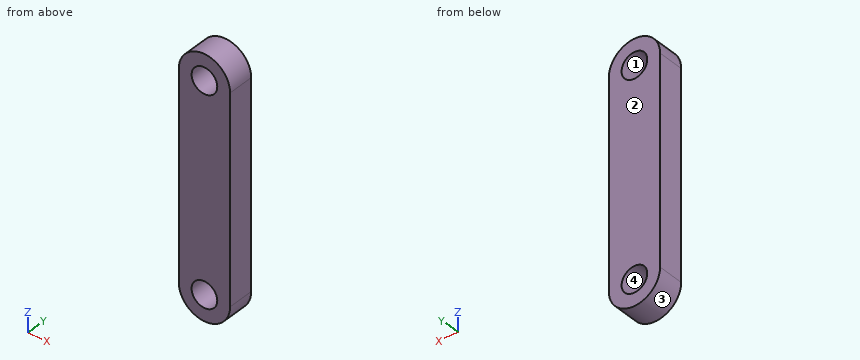
```python
from build123d import *

# Parameters (mm, degrees)
F0_R     = 3.75
F1_DEPTH = 7.62


with BuildPart() as f1:
    # F0 (on Front) → F1 (new body)
    with BuildSketch(Plane.XZ):
        with BuildLine():
            Line((7.5, 0), (7.5, 60))
            ThreePointArc((7.5, 60), (0, 52.5), (-7.5, 60))
            Line((-7.5, 60), (-7.5, 0))
            ThreePointArc((-7.5, 0), (0, 7.5), (7.5, 0))
        make_face()
        with BuildLine():
            ThreePointArc((-7.5, 60), (0, 52.5), (7.5, 60))
            ThreePointArc((7.5, 60), (0, 67.5), (-7.5, 60))
        make_face()
        with Locations((0, 60)):
            Circle(F0_R, mode=Mode.SUBTRACT)
        with BuildLine():
            ThreePointArc((-7.5, 0), (0, -7.5), (7.5, 0))
            ThreePointArc((7.5, 0), (0, 7.5), (-7.5, 0))
        make_face()
        Circle(F0_R, mode=Mode.SUBTRACT)
    extrude(amount=F1_DEPTH)


solid = f1.part
```
Could you check a few things on this model? Use its own coordinates, in mm. Face numbers are marked on the shaded views. Coordinates: 2 decimals unless noted, no trailing zeros. Loops run counter-clockwise (first coordinate to the right, second up) from the corner with the lowest first, then second, coordinate; pieces in that order, holes last. Notation, with made-up numbers: M 48,13.5 L 78,13.5 A25 ccw 78,37.5 Z; hole C 65,40 d2. An arc over 180 degrees is marked long. Put each result on its own line as item: value. Start each with the question number.
(1) Suppose I cut it at C-C on x = -6. Please give me the cut outline in (y, z).
(2) Thinking about a two-plate mould opening in Z: for the marked faces 1, 2, 3 and 4, which applies, pulls with the +Z half, pulls with the -Z half, needs draft (parallel to the pull), parting line crosses it, or undercut?
(3) Will these pins go through, and if not, where does the flat tip stop? P1, Ø2, axis at x = -5.5, y = -6.5, coming from the -Z side; P2, Ø1, axis at x = -1, y = -6, coming from the -Z side.
(4) Suppose I cut it at A-A on x = 0. Please give me the cut outline in (y, z).
(5) I need wall thicknesses on line 1 (Z direction, x = 0, y = -2); line 2 (Z direction, x = 1.5, y = -2.5); line 3 (X direction, y = -1.5, z = 3). Which ranges of each line are inside material? Lowest first, please. Write a range as from..to.
(6) Suppose I cut it at B-B on y = -6.75. Please give me the cut outline in (x, z).
Solutions:
1. outline: M -7.62,-4.5 L 0,-4.5 L 0,64.5 L -7.62,64.5 Z
2. face 1: undercut
2. face 2: needs draft
2. face 3: pulls with the -Z half
2. face 4: undercut
3. P1: stops at z = -6
3. P2: stops at z = -7.48
4. outline: M -7.62,-7.5 L 0,-7.5 L 0,-3.75 L -7.62,-3.75 Z; M -7.62,3.75 L 0,3.75 L 0,56.25 L -7.62,56.25 Z; M -7.62,63.75 L 0,63.75 L 0,67.5 L -7.62,67.5 Z
5. line 1: z = -7.5..-3.75, 3.75..56.25, 63.75..67.5
5. line 2: z = -7.35..-3.44, 3.44..56.56, 63.44..67.35
5. line 3: x = -7.5..-2.25, 2.25..7.5
6. outline: M -7.5,0 A7.5 ccw 7.5,0 L 7.5,60 A7.5 ccw -7.5,60 Z; hole C 0,0 d7.5; hole C 0,60 d7.5
